Verification items for this drawing (mm, ordinates from the low corner). Round coordinates to 2 decimals unless told otherwise and drop trailing zeros. Loops run counter-clockwise (first coordinate to the right, second up) from the corner with the lowest first, then second, coordinate; pieces in that order, holes last. Notation, with made-up numbers: (-20.5, 33) - (14.5, 33) arc R17 ccw to (14.5, 42) - close; hole circle Ø10 at (21, 39.25). An arc over 180 degrees is marked (long way). Write item = value, one per line.
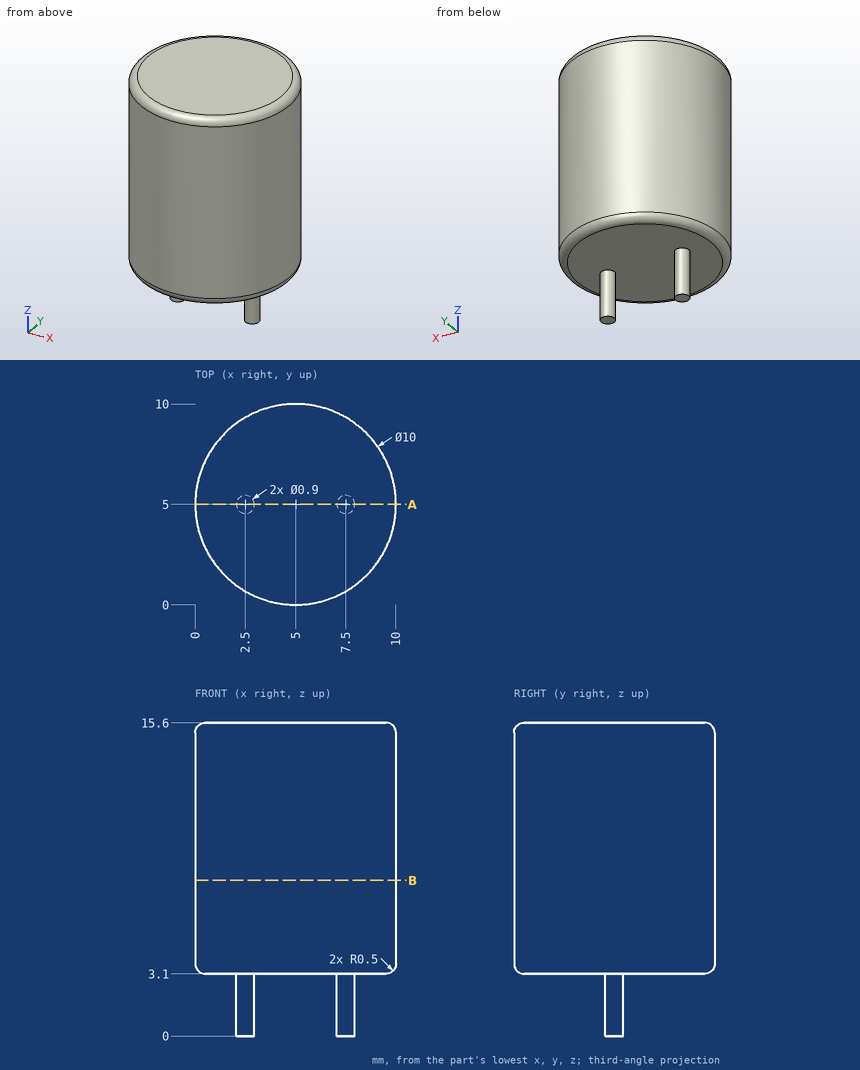
(1) Section check B-B (z = 7.75). Enter the section's corners in (x, y).
Answers follow:
outline = circle Ø10 at (5, 5)
(2) Gauge pin test, flat ends, axial feed: pin 1 (1.5 mm diameter, centred on x = 3, y = 3, fed in from -Z); pin 2 (1 mm diameter, centred on y = 2, z = 1.5, fed in from +X); pin 3 (3 mm diameter, centred on y = 9, z = 5.5, fed in from -X); pin 4 (5 mm diameter, centred on y = 3, z = 2.5, fed in from +X). Record the tip position at first contact, or that the pin passes through.
Answers follow:
pin_1 = 3.1
pin_2 = through
pin_3 = 0.67
pin_4 = 10
(3) Section check A-A (y = 5). Enter the section's corners in (x, z).
Answers follow:
outline = (0, 3.6) arc R0.5 ccw to (0.5, 3.1) - (2.05, 3.1) - (2.05, 0) - (2.95, 0) - (2.95, 3.1) - (7.05, 3.1) - (7.05, 0) - (7.95, 0) - (7.95, 3.1) - (9.5, 3.1) arc R0.5 ccw to (10, 3.6) - (10, 15.1) arc R0.5 ccw to (9.5, 15.6) - (0.5, 15.6) arc R0.5 ccw to (0, 15.1) - close
(4) Scan lines: L1, parallel to Z at x = 9, y = 5.75; L2, parallel to X at y = 9.25, z = 12; L3, parallel to X at y = 3.75, z = 14.5. Record each from-to range of solid material in increasing order. Write a range as [from, to].
Answers follow:
L1 = [3.1, 15.6]
L2 = [2.37, 7.63]
L3 = [0.16, 9.84]
